Build history of the part. All positions in model axes, mm. Face numbers are marked on the shaded views. A direction names the side the tool comes from. Round coordinates to 2 decimals unless told otherwise and drop trailing zeros. Write each loop counter-clockwise with the first axis right and the second up, starting at its lowest first coordinate (ties: lowest second). Pieces come first, ordered by that corner, then holes. Notation, with made-up numbers: (76, 84) - (83, 84) arc R19 cw to (83, 94) - close; hole circle Ø7 at (-37.75, 70.5). An arc over 180 degrees is marked (long way). Write each question's results on one line, items separated by ' | '.
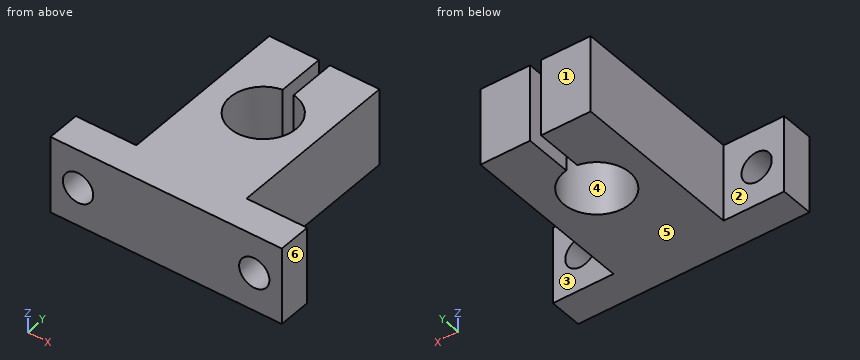
Autodesk Inventor part; units mm, degrees
ref_plane "YZ Plane" through (0, 0, 0) normal (1, 0, 0) x (0, 1, 0)
ref_plane "XZ Plane" through (0, 0, 0) normal (0, 1, 0) x (-1, 0, 0)
ref_plane "XY Plane" through (0, 0, 0) normal (0, 0, 1) x (1, 0, 0)
sketch "Sketch1" plane through (0, 0, 0) normal (0, 0, 1) x (1, 0, 0)
  arc A0 (-1, 5.9161) -> (1, 5.9161) centre (0, 0) ccw
  line L0 (-21, -23) -> (21, -23)
  line L1 (-21, -23) -> (-21, -17)
  line L2 (21, -23) -> (21, -17)
  line L3 (-10, 14.5) -> (-10, -17)
  line L4 (-10, -17) -> (-21, -17)
  line L5 (-10, 14.5) -> (-1, 14.5)
  line L6 (10, 14.5) -> (1, 14.5)
  line L7 (1, 14.5) -> (1, 5.9161)
  line L8 (-1, 14.5) -> (-1, 5.9161)
  line L9 (10, 14.5) -> (10, -17)
  line L10 (10, -17) -> (21, -17)
  dimension "d0" = 12
  dimension "d1" = 23
  dimension "d2" = 42
  dimension "d3" = 21
  dimension "d4" = 6
  dimension "d7" = 9
  dimension "d8" = 9
  dimension "d10" = 37.5
  dimension "d11" = 37.5
  dimension "d14" = 10
  dimension "d15" = 31.5
  dimension "d16" = 6
  dimension "d17" = 10
extrude "Extrusion1" add sketch "Sketch1" along normal blind 14
sketch "Sketch2" plane through (10, -17, 0) normal (0, 1, 0) x (1, 0, 0)
  circle A0 centre (-26, -7) radius 2.75
  circle A1 centre (6, -7) radius 2.75
  line L0 (-10, 2.8) -> (-10, -16.8)
  line L1 (-20, -14) -> (-31, -14)
  point P0 (-10, 0)
  dimension "d20" = 5.5
  dimension "d21" = 5.5
  dimension "d22" = 32
  dimension "d23" = 16
  dimension "d24" = 7
  dimension "d25" = 16
extrude "Extrusion2" cut sketch "Sketch2" against normal blind 14
properties part number "SK12"
(1) Slice it at C-C, the plane y = 10.5. Write the cut outline in (x, z).
Worked answers:
outline: (-10, 0) - (-1, 0) - (-1, 14) - (-10, 14) - close; (1, 0) - (10, 0) - (10, 14) - (1, 14) - close
(2) Slice it at A-A, the plane x = 16. Write the cut outline in (y, z), and give its area (3 significant figures).
Worked answers:
outline: (-23, 0) - (-17, 0) - (-17, 4.25) - (-23, 4.25) - close; (-23, 9.75) - (-17, 9.75) - (-17, 14) - (-23, 14) - close | area: 51.0 mm2
(3) Two-plate mould, pull along X, no slides. Class the marked faces 4, 5 and 6: released by +X, released by -X, zero draft, split by the parting line, or undercut.
Worked answers:
face 4: undercut | face 5: zero draft | face 6: released by +X
(4) Flat gauge pins, fed straight in: pin 1 Ø10 at (x, y) = (-6, -18) entering from -Z; pin 2 Ø7 at (y, z) = (10.5, 7.5) entering from -X; pin 3 Ø6 at (y, z) = (9, 7) entering from +X; pin 4 Ø3.5 at (x, z) = (-16, 5.5) entering from +Y. Where does each tip first touch, or does it go through?
Worked answers:
pin 1: stops at z = 0 | pin 2: stops at x = -10 | pin 3: stops at x = 10 | pin 4: stops at y = -17
(5) Slice it at B-B, the plane z = 7. Write the cut outline in (x, y), and give its area (3 significant figures).
Worked answers:
outline: (-21, -23) - (-18.75, -23) - (-18.75, -17) - (-21, -17) - close; (-13.25, -23) - (13.25, -23) - (13.25, -17) - (10, -17) - (10, 14.5) - (1, 14.5) - (1, 5.92) arc R6 cw (long way) to (-1, 5.92) - (-1, 14.5) - (-10, 14.5) - (-10, -17) - (-13.25, -17) - close; (18.75, -23) - (21, -23) - (21, -17) - (18.75, -17) - close | area: 686 mm2
(6) Tool access for the marked faces 1, 2 and 3: list every direction of +Z, -Z, +X, -X, +Y, -Y with a clear straight run to the whole face (end or side of a thin tool).
Worked answers:
face 1: +Z, -Z, +X, -X, +Y | face 2: +Z, -Z, -X, +Y | face 3: +Z, -Z, +X, +Y
(7) Slice it at D-D, the plane x = 0. Write the cut outline in (y, z), and give its area (3 significant figures).
Worked answers:
outline: (-23, 0) - (-6, 0) - (-6, 14) - (-23, 14) - close | area: 238 mm2
(8) Drill centre lines: probe 1 along X at (y, z) = (-18.85, 7); probe 2 along X at (y, z) = (13.5, 4.75); probe 3 along X at (y, z) = (0, 8). Where is each one in solid material? Low to high. Write a range as [from, to].
Worked answers:
probe 1: x = [-21, -18.75], [-13.25, 13.25], [18.75, 21] | probe 2: x = [-10, -1], [1, 10] | probe 3: x = [-10, -6], [6, 10]
